Part print with two shaded views. Sizes in mm from the minimum x, y, z corner. Round coordinates to 2 decimals unless told otherwise and drop trailing zeros. Order: outer loops, then holes, each group sorted by start corner. A loop starts at its lowest first (then second) coordinate and runs counter-clockwise, first axis right, second up. Notation, with made-up numbers: (-26, 27.5) -> (32, 27.5) arc R13 ccw to (32, 41.5) -> close; hole circle Ø4 at (-2, 62.5). An arc over 180 degrees is marked (long way). Answer as a JSON object with one key per item and string values.
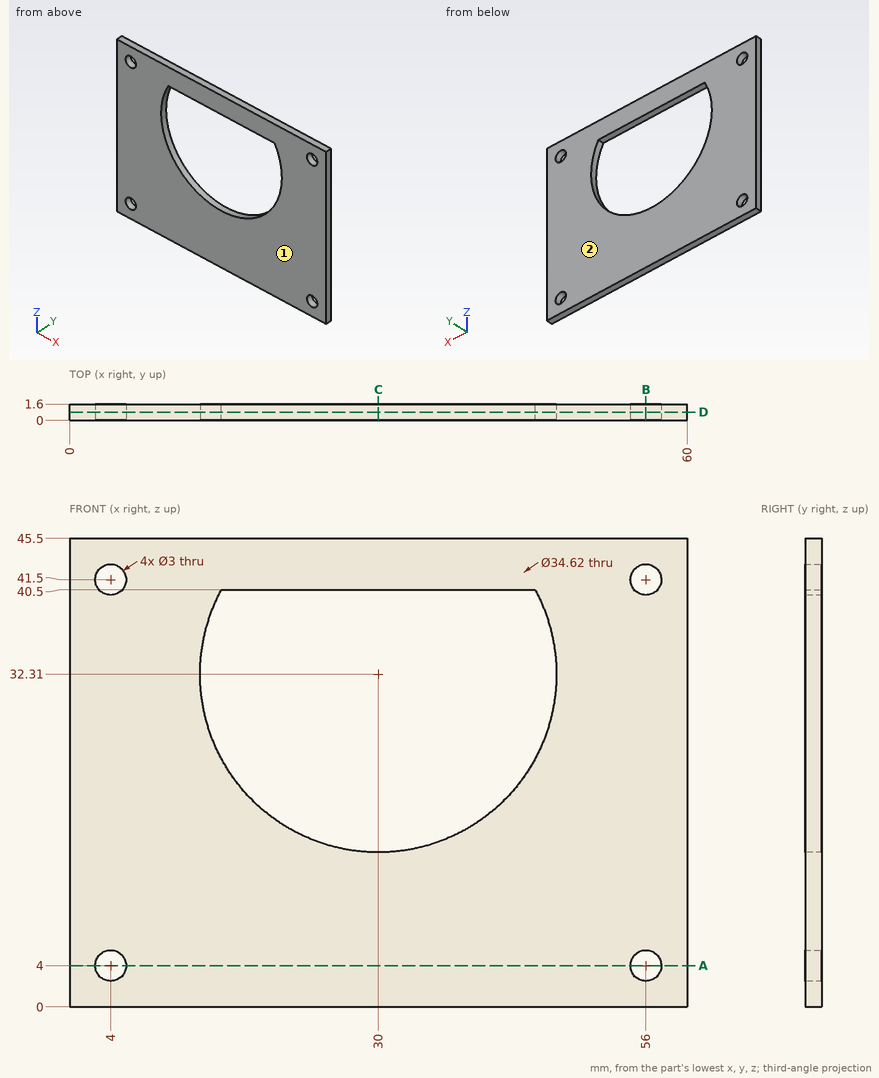
1) Pull direction Y, two halves, no side cores. Call the marked faces 1 and 2: pulls with the +Y half, pulls with the -Y half, needs draft (parallel to the pull), parting line crosses it, or undercut.
Checked values:
{"face 1": "pulls with the -Y half", "face 2": "pulls with the +Y half"}
2) Cut at A-A, the plane z = 4. Give the cut face in (x, y), plus the area to 3 significant figures.
Checked values:
{"outline": "(0, 0) -> (2.5, 0) -> (2.5, 1.6) -> (0, 1.6) -> close; (5.5, 0) -> (54.5, 0) -> (54.5, 1.6) -> (5.5, 1.6) -> close; (57.5, 0) -> (60, 0) -> (60, 1.6) -> (57.5, 1.6) -> close", "area": "86.4 mm²"}
3) Cut at C-C, the plane x = 30. Give the cut face in (y, z), plus the area to 3 significant figures.
Checked values:
{"outline": "(0, 0) -> (1.6, 0) -> (1.6, 15) -> (0, 15) -> close; (0, 40.5) -> (1.6, 40.5) -> (1.6, 45.5) -> (0, 45.5) -> close", "area": "32.0 mm²"}
4) Cut at B-B, the plane x = 56. Give the cut face in (y, z).
Checked values:
{"outline": "(0, 0) -> (1.6, 0) -> (1.6, 2.5) -> (0, 2.5) -> close; (0, 5.5) -> (1.6, 5.5) -> (1.6, 40) -> (0, 40) -> close; (0, 43) -> (1.6, 43) -> (1.6, 45.5) -> (0, 45.5) -> close"}
5) Probe L1, parallel to X at y = 0.7, z = 4; L2, parallel to Z at x = 29.5, y = 0.9; L3, parallel to X at y = 1.25, z = 33. List the from-to ranges inside material, lowest first. Write a range as from..to.
Checked values:
{"L1": "x = 0..2.5, 5.5..54.5, 57.5..60", "L2": "z = 0..15.01, 40.5..45.5", "L3": "x = 0..12.7, 47.3..60"}
6) Flat gauge pin, fed straight in: pin 1 Ø3.5 at (x, z) = (56, 4) entering from -Y. Where does the tip first touch, or does it go through?
Checked values:
{"pin 1": "stops at y = 0"}
7) Cut at D-D, the plane y = 0.8. Give the cut face in (x, z), plus the area to 3 significant figures.
Checked values:
{"outline": "(0, 0) -> (60, 0) -> (60, 45.5) -> (0, 45.5) -> close; hole circle Ø3 at (4, 4); hole circle Ø3 at (4, 41.5); hole (14.75, 40.5) arc R17.31 ccw (long way) to (45.25, 40.5) -> close; hole circle Ø3 at (56, 4); hole circle Ø3 at (56, 41.5)", "area": "1,960 mm²"}
